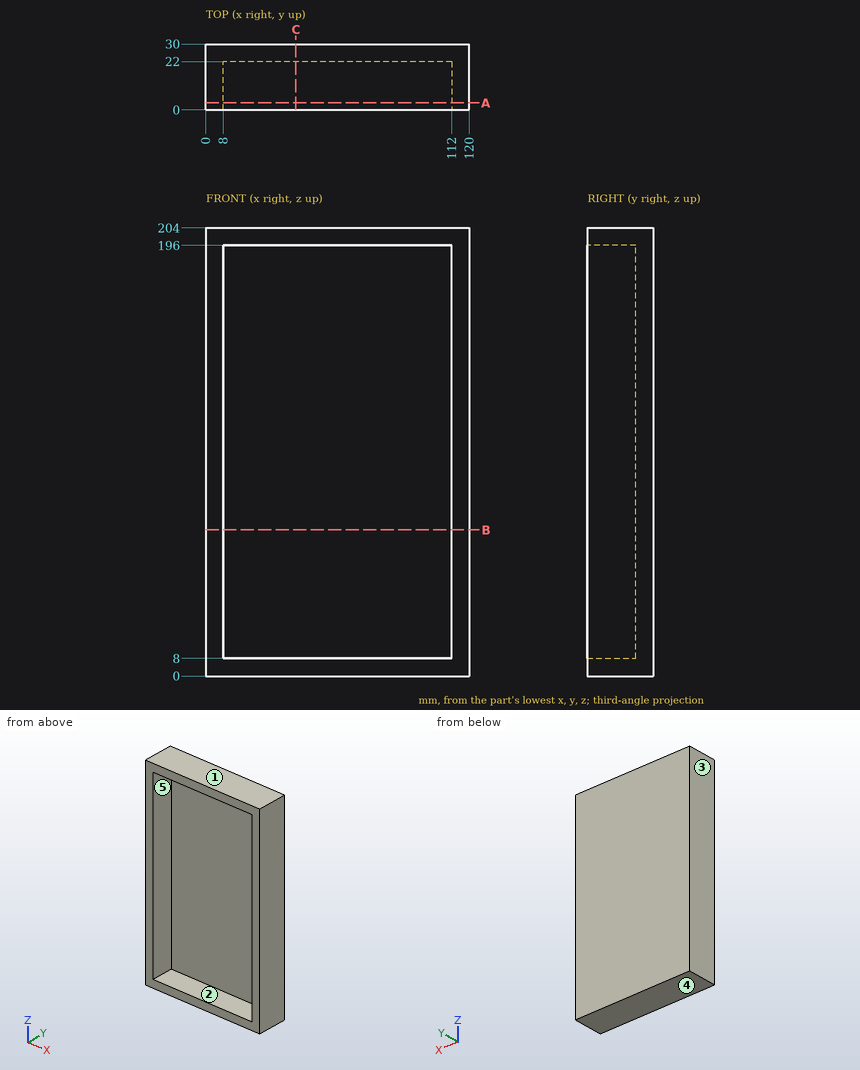
Source: three-view drawing plus pictorial views. Frame: mm from the lowest corner of the part. A direction names the side the tool comes from. Coordinates: 2 decimals unless noted, no trailing zeros. Loops run counter-clockwise (first coordinate to the right, second up) from the corner with the lowest first, then second, coordinate; pieces in that order, holes last. Notation, with made-up numbers: (62.25, 22) - (78.25, 22) arc R17 ccw to (78.25, 41) - close; hole circle Ø5 at (9.25, -34). An arc over 180 degrees is marked (long way). Answer in a Markdown table with one row per item. Add a question column.
Item 1: Mould query, pull axis Z, two halves, no side actions, for the marked faces 3, 4 and 5. Classes: released by +Z, released by -Z, zero draft, split by the parting line, or undercut.
Item 2: Access query for the marked faces 1 and 2. Directions: +Z, -Z, +X, -X, +Y, -Y. A direction counts if a zero-diameter tool reaches every point of the face in a straight line with its end or side. Return the directions, or none.
Item 3: Contact query for a flat-ended pin moving along its axis: P1, Ø12, axis at x = 36.5, z = 160, coming from the -Y side. Output: stop coordinate, or through.
Item 4: Section query A-A on y = 3.25. Return the cut outline in (x, z), then the cut area to 3 significant figures.
Item 5: Section query B-B on z = 66.5. Return the cut outline in (x, y).
Item 6: Section query C-C on x = 41. Return the cut outline in (y, z), then the cut area to 3 significant figures.
Item 7: Line query: line 1 along X through (y, z) = (11, 33); line 2 along Z through (x, y) = (87, 10.5); line 3 along Y through (x, z) = (20.5, 44.5). Output: solid intervals per line, ascending. Write a range as [from, to].
Recorded:
| question | item | result |
|---|---|---|
| 1 | face 3 | zero draft |
| 1 | face 4 | released by -Z |
| 1 | face 5 | undercut |
| 2 | face 1 | +Z, +X, -X, +Y, -Y |
| 2 | face 2 | -Y |
| 3 | P1 | y = 22 |
| 4 | outline | (0, 0) - (120, 0) - (120, 204) - (0, 204) - close; hole (8, 8) - (112, 8) - (112, 196) - (8, 196) - close |
| 4 | area | 4,930 mm^2 |
| 5 | outline | (0, 0) - (8, 0) - (8, 22) - (112, 22) - (112, 0) - (120, 0) - (120, 30) - (0, 30) - close |
| 6 | outline | (0, 0) - (30, 0) - (30, 204) - (0, 204) - (0, 196) - (22, 196) - (22, 8) - (0, 8) - close |
| 6 | area | 1,980 mm^2 |
| 7 | line 1 | [0, 8], [112, 120] |
| 7 | line 2 | [0, 8], [196, 204] |
| 7 | line 3 | [22, 30] |
